Build history of the part. All positions in model axes, mm. A direction names the side the tool comes from. Coordinates: 2 decimals unless noted, no trailing zeros. Loops run counter-clockwise (first coordinate to the right, second up) from the corner with the lowest first, then second, coordinate; pieces in that order, holes last.
Item 1: Flat gauge pins, fed straight in: pin 1 (1.5 mm diameter, centred on x = 39, z = 23, fed in from +Y); pin 2 (1.4 mm diameter, centred on x = 52, y = 40, fed in from -Z); pin 3 (1.6 mm diameter, centred on x = 45, z = 27, fed in from -Y). Where does each tip first touch, or does it go through?
Item 2: 3-axis set-ups, long thin cutter, end or side, ignore diameter. For faces 1 (the face through (52, 22, 22.5)), 2 (the face through (2.5, 25, -12)), 3 (the face through (25, 25, 55)), 4 (the face through (52, 17.5, 27)), 5 (the face through (53, 40, 26.086)): which of +Z, -Z, +X, -X, +Y, -Y reach the whole face in a straight line?
Item 3: Drill centre lines: line 1 along Y through (x, z) = (17, 44); line 2 along Y through (x, z) = (27, -16.5); line 3 along X through (y, z) = (49, 27.5). Where is each one in solid material? Low to high.
Item 4: Cut at D-D (x = 25.5). List the corners of the cut face in (y, z), and give its area (3 significant figures).
Item 5: Cut at C-C (z = -9). List the corners of the cut face in (x, y).
Item 6: Mould opens along Y. For faces 6 (the face through (25, 45, 16)), 7 (the face through (25, 47.5, -12)), 8 (the face through (53, 40, 28.661)), 9 (the face through (25, 2.5, -12)) say: released by +Y, released by -Y, zero draft, split by the parting line, or undercut.
Item 7: Cut at B-B (y = 43.5). List the corners of the cut face in (x, z).
Item 8: Cut at A-A (x = 46). List the corners of the cut face in (y, z), and give its area (3 significant figures).
from build123d import *

# Parameters (mm, degrees)
F0_W      = 50
F0_H      = 50
F0_W_2    = 40
F0_H_2    = 40
F1_DEPTH  = 55
F2_W      = 55
F2_H      = 55
F3_DEPTH  = 5
F4_W      = 45
F4_H      = 45
F4_W_2    = 40
F4_H_2    = 40
F5_DEPTH  = 25
F6_W      = 10
F6_H      = 10
F7_DEPTH  = 5
F8_W      = 2
F8_H      = 2
F9_DEPTH  = 25
F11_W     = 10
F11_H     = 10
F12_DEPTH = 5
F13_W     = 2.745383
F13_H     = 2.574146
F14_DEPTH = 25


with BuildPart() as f1:
    # F0 (on Top) → F1 (new body)
    with BuildSketch(Plane.XY):
        with Locations((25, 25)):
            Rectangle(F0_W, F0_H)
        with Locations((25, 25)):
            Rectangle(F0_W_2, F0_H_2, mode=Mode.SUBTRACT)
    extrude(amount=F1_DEPTH)

    # F2 (on face) → F3 (join)
    with BuildSketch(Plane.XY.offset(55)):
        with Locations((25, 25)):
            Rectangle(F2_W, F2_H)
    extrude(amount=F3_DEPTH)

    # F4 (on face) → F5 (join)
    with BuildSketch(Plane(origin=(0, 0, 0), x_dir=(1, 0, 0), z_dir=(0, 0, -1))):
        with Locations((25, -25)):
            Rectangle(F4_W, F4_H)
        with Locations((25, -25)):
            Rectangle(F4_W_2, F4_H_2, mode=Mode.SUBTRACT)
    extrude(amount=F5_DEPTH)

    # F6 (on face) → F7 (join)
    with BuildSketch(Plane(origin=(0, 50, 0), x_dir=(-1, 0, 0), z_dir=(0, 1, 0))):
        with Locations((-25, 27.5)):
            Rectangle(F6_W, F6_H)
    extrude(amount=F7_DEPTH)

    # F8 (on face) → F9 (join)
    with BuildSketch(Plane.YZ.offset(30)):
        with Locations((52.5, 27.5)):
            Rectangle(F8_W, F8_H)
    extrude(amount=F9_DEPTH)

    # F11 (on face) → F12 (join)
    with BuildSketch(Plane.YZ.offset(50)):
        with Locations((22.5, 27.5)):
            Rectangle(F11_W, F11_H)
    extrude(amount=F12_DEPTH)

    # F13 (on face) → F14 (join)
    with BuildSketch(Plane(origin=(0, 27.5, 0), x_dir=(-1, 0, 0), z_dir=(0, 1, 0))):
        with Locations((-52.646901, 27.373498)):
            Rectangle(F13_W, F13_H)
    extrude(amount=F14_DEPTH)


solid = f1.part
Filled sheet:
1. pin 1: stops at y = 50
1. pin 2: stops at z = 26.09
1. pin 3: stops at y = 0
2. face 1: -Z, +X, +Y, -Y
2. face 2: -Z, -X, +Y, -Y
2. face 3: -Z
2. face 4: -Z, +X, -Y
2. face 5: -Z, +X, +Y
3. line 1: y = 0 to 5, 45 to 50
3. line 2: y = 2.5 to 5, 45 to 47.5
3. line 3: x = 0 to 50, 51.27 to 54.02
4. outline: (-2.5, 55) - (0, 55) - (0, 0) - (2.5, 0) - (2.5, -25) - (5, -25) - (5, 55) - (45, 55) - (45, -25) - (47.5, -25) - (47.5, 0) - (50, 0) - (50, 22.5) - (55, 22.5) - (55, 32.5) - (50, 32.5) - (50, 55) - (52.5, 55) - (52.5, 60) - (-2.5, 60) - close
4. area: 1,000 mm2
5. outline: (2.5, 2.5) - (47.5, 2.5) - (47.5, 47.5) - (2.5, 47.5) - close; hole (5, 5) - (45, 5) - (45, 45) - (5, 45) - close
6. face 6: undercut
6. face 7: released by +Y
6. face 8: zero draft
6. face 9: released by -Y
7. outline: (-2.5, 55) - (0, 55) - (0, 0) - (2.5, 0) - (2.5, -25) - (5, -25) - (5, 55) - (45, 55) - (45, -25) - (47.5, -25) - (47.5, 0) - (50, 0) - (50, 55) - (52.5, 55) - (52.5, 60) - (-2.5, 60) - close; (51.27, 26.09) - (54.02, 26.09) - (54.02, 28.66) - (51.27, 28.66) - close
8. outline: (-2.5, 55) - (0, 55) - (0, 0) - (2.5, 0) - (2.5, -25) - (47.5, -25) - (47.5, 0) - (50, 0) - (50, 55) - (52.5, 55) - (52.5, 60) - (-2.5, 60) - close; (51.5, 26.5) - (53.5, 26.5) - (53.5, 28.5) - (51.5, 28.5) - close
8. area: 4,150 mm2
